The figure shows three views and two pictorial views of one solid part (mm, origin at its lowest corner). Answer the questions. A direction names the side the tool comes from. Give positions to 0.01 mm unless a question says otherwise; leave off trailing zeros. Write each loop counter-clockwise with the first axis right and the second up, starting at its lowest first coordinate (ties: lowest second). Pieces come first, ordered by that corner, then holes. Notation, with made-up numbers: (-22.75, 32) - (21.25, 32) arc R20 ccw to (21.25, 36) - close; hole circle Ø7 at (-36, 1). An arc over 180 degrees is marked (long way). One line per question, with ' | ' between items. Start each with the question number.
1. A cutting plane is placed at D-D (z = 103). Determine the outline of the cut face in (x, y).
2. A cutting plane is placed at A-A (y = 40). Determine the outline of the cut face in (x, z).
3. For the marked faces 5, 6 and 7, determine the directions among +Z, -Z, +X, -X, +Y, -Y from which every point of the face is accessible in a straight line to the end or side of a thin tool.
4. A cutting plane is placed at B-B (y = 27.5). Determine the outline of the cut face in (x, z).
5. A cutting plane is placed at C-C (y = 13). Determine the outline of the cut face in (x, z).
6. The mould has two halves that part along Z. Classify the marked faces 1, 2, 3 and 4: +Z half, -Z half, draft (parallel to the pull), parting line (faces both ways), or undercut.
7. Find the intervals of material crossed by L1, parallel to Z at x = 70, y = 27; L2, parallel to Y at x = 16, z = 50; L3, parallel to X at y = 72, z = 88, in increasing order. Write a range as from..to.
8. Given P1, Ø8, axis at x = 68.5, z = 33.5, coming from the +Y side; P2, Ø5, axis at x = 86, y = 13.5, coming from the -Z side; P3, Ø9.5, axis at x = 69, z = 90.5, coming from the +Y side, each flat-ended and moving along its own axis, determine where each tip first touches the part or whether it passes through.
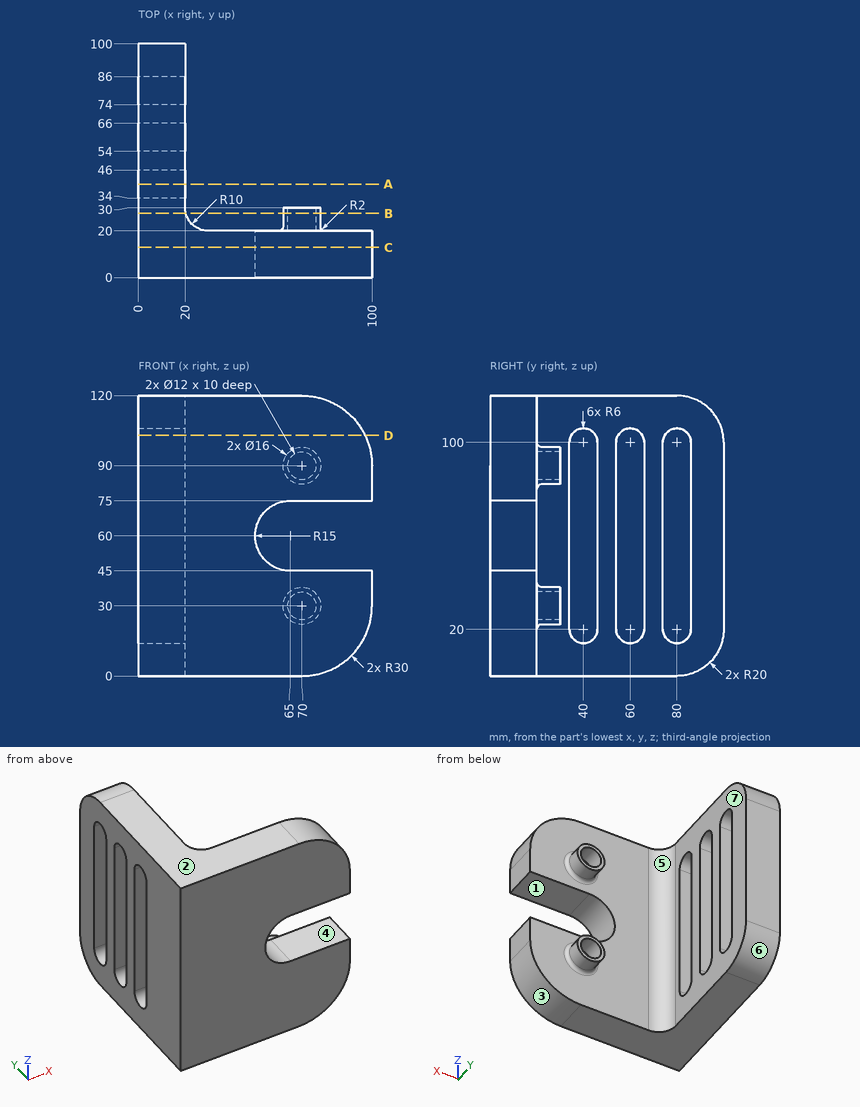
Determined:
1) outline: (0, 0) - (97.04, 0) - (97.04, 20) - (30, 20) arc R10 cw to (20, 30) - (20, 34.8) - (0, 34.8) - close; (0, 45.2) - (20, 45.2) - (20, 54.8) - (0, 54.8) - close; (0, 65.2) - (20, 65.2) - (20, 74.8) - (0, 74.8) - close; (0, 85.2) - (20, 85.2) - (20, 99.77) - (0, 99.77) - close
2) outline: (0, 0) - (20, 0) - (20, 14) - (0, 14) - close; (0, 106) - (20, 106) - (20, 120) - (0, 120) - close
3) face 5: +Z, -Z, +Y | face 6: -Z, +X, -X, +Y | face 7: +Z, -Z, +X, +Y
4) outline: (0, 0) - (20.32, 0) - (20.32, 120) - (0, 120) - close; circle Ø16 at (70, 30); circle Ø16 at (70, 90); hole circle Ø12 at (70, 30); hole circle Ø12 at (70, 90)
5) outline: (0, 0) - (70, 0) arc R30 ccw to (100, 30) - (100, 45) - (65, 45) arc R15 cw to (65, 75) - (100, 75) - (100, 90) arc R30 ccw to (70, 120) - (0, 120) - close
6) face 1: undercut | face 2: +Z half | face 3: -Z half | face 4: undercut
7) L1: 22..24, 36..38, 82..84, 96..98 | L2: 0..34, 46..54, 66..74, 86..100 | L3: 0..20
8) P1: y = 30 | P2: z = 3.21 | P3: y = 20
